The model under review builds one solid part; all positions refer to its coordinate system, in mm. Face numbers are marked on the shaded views. A direction names the side the tool comes from. Round coordinates to 2 decimals unless told otherwise and drop trailing zeros. Order: outer loops, then holes, each group sorted by start corner. A loop starts at its lowest first (then second) coordinate and runs counter-clockwise, first axis right, second up.
1) Machinability: for the marked faces 1, 2 and 3, which of the approach directions +Z, -Z, +X, -X, +Y, -Y give a long, thin tool a straight path to every point of the face, cutting with its end or side? Answer none if there is none.
2) Mouldability with a two-part tool opening along X and no side actions: class the marked faces 4, 5 and 6 as pulls with the +X half, pulls with the -X half, needs draft (parallel to the pull), parting line crosses it, or undercut.
3) Consider section D-D (x = -28.5). Give the boundary of the cut face in (y, z), then the cut area to 3 significant figures.
4) Clearance check with flat-ended pins moving along their axes: P1, Ø1, axis at y = -8, z = -7.5, coming from the +X side (3 decimals); P2, Ø12, axis at x = -48.5, z = -2.5, coming from the +Y side; P3, Ø3.5, axis at y = -9.5, z = -0.5, coming from the -X side (3 decimals). State where each tip first meets the part, or that it passes through.
5) To check wall thickness, follow L1, parallel to X at y = -9.25, z = 2.75 (3 decimals); L2, parallel to X at y = -0.2, z = 0 (3 decimals); L3, parallel to Y at x = 38, z = -1.25. State the ranges of each line that lie inside material, in increasing order.
6) Consider section A-A (z = 0). Give the boundary of the cut face in (x, y) (3 decimals).
7) Consider section B-B (y = -7). Give the boundary of the cut face in (x, z) (3 decimals).
8) Consider section C-C (z = -4.5). Give the boundary of the cut face in (x, y) (3 decimals).
from build123d import *

# Parameters (mm, degrees)
SKETCH1_W          = 82.55
SKETCH1_H          = 25.4
BASE_FLANGE1_DEPTH = 0.7
EDGE_FLANGE1_DEPTH = 25.4
EDGE_FLANGE2_DEPTH = 25.4
EDGE_FLANGE3_DEPTH = 25.4
EDGE_FLANGE4_DEPTH = 25.4
SKETCH19_R         = 2.35
CUT_EXTRUDE1_DEPTH = 59.231440176


# Sheet-metal steps are written as plain solids
with BuildPart() as part:
    # Sketch1 → Base-Flange1 (new body)
    with BuildSketch(Plane(origin=(0, 0, 0), x_dir=(1, 0, 0), z_dir=(0, 1, 0))):
        Rectangle(SKETCH1_W, SKETCH1_H)
    extrude(amount=-BASE_FLANGE1_DEPTH)

    # Edge-Flange1 section (across the edge) → Edge-Flange1 (add)
    with BuildSketch(Plane(origin=(42.275, -0.7, -12.7), x_dir=(-1, 0, 0), z_dir=(0, 0, 1))):
        with BuildLine():
            Line((-0.7, 1), (-0.7, 12))
            Line((-0.7, 12), (0, 12))
            Line((0, 12), (0, 1))
            ThreePointArc((0, 1), (0.292893219, 0.292893219), (1, 0))
            Line((1, 0), (1, -0.7))
            ThreePointArc((1, -0.7), (-0.202081528, -0.202081528), (-0.7, 1))
        make_face()
    extrude(amount=EDGE_FLANGE1_DEPTH)

    # Edge-Flange2 section (across the edge) → Edge-Flange2 (add)
    with BuildSketch(Plane(origin=(42.975, -13.7, 12.7), x_dir=(0, 1, 0), z_dir=(0, 0, -1))):
        with BuildLine():
            Line((-0.7, 1), (-0.7, 12))
            Line((-0.7, 12), (0, 12))
            Line((0, 12), (0, 1))
            ThreePointArc((0, 1), (0.292893219, 0.292893219), (1, 0))
            Line((1, 0), (1, -0.7))
            ThreePointArc((1, -0.7), (-0.202081528, -0.202081528), (-0.7, 1))
        make_face()
    extrude(amount=EDGE_FLANGE2_DEPTH)

    # Edge-Flange3 section (across the edge) → Edge-Flange3 (add)
    with BuildSketch(Plane(origin=(-42.275, -0.7, 12.7), x_dir=(1, 0, 0), z_dir=(0, 0, -1))):
        with BuildLine():
            Line((-0.7, 1), (-0.7, 12))
            Line((-0.7, 12), (0, 12))
            Line((0, 12), (0, 1))
            ThreePointArc((0, 1), (0.292893219, 0.292893219), (1, 0))
            Line((1, 0), (1, -0.7))
            ThreePointArc((1, -0.7), (-0.202081528, -0.202081528), (-0.7, 1))
        make_face()
    extrude(amount=EDGE_FLANGE3_DEPTH)

    # Edge-Flange4 section (across the edge) → Edge-Flange4 (add)
    with BuildSketch(Plane(origin=(-42.975, -13.7, -12.7), x_dir=(0, 1, 0), z_dir=(0, 0, 1))):
        with BuildLine():
            Line((-0.7, 1), (-0.7, 12))
            Line((-0.7, 12), (0, 12))
            Line((0, 12), (0, 1))
            ThreePointArc((0, 1), (0.292893219, 0.292893219), (1, 0))
            Line((1, 0), (1, -0.7))
            ThreePointArc((1, -0.7), (-0.202081528, -0.202081528), (-0.7, 1))
        make_face()
    extrude(amount=EDGE_FLANGE4_DEPTH)

    # Sketch19 → Cut-Extrude1 (cut, through all)
    with BuildSketch(Plane(origin=(0, 0, 0), x_dir=(1, 0, 0), z_dir=(0, 1, 0))):
        with Locations(Location((-33.3248, 0, 0), (0, 0, 270))):
            Circle(SKETCH19_R)
        with Locations(Location((3.175, 0, 0), (0, 0, 270))):
            Circle(SKETCH19_R)
    extrude(amount=-CUT_EXTRUDE1_DEPTH, mode=Mode.SUBTRACT)


solid = part.part
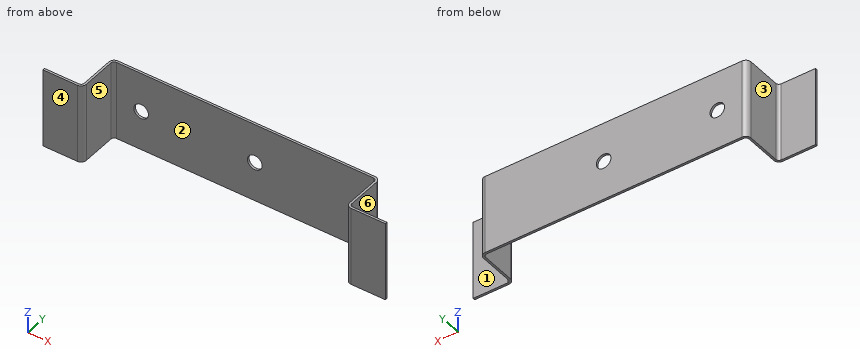
Answer below:
1. face 1: +Z, -Z, +X, +Y
1. face 2: +Z, -Z, -Y
1. face 3: +Z, -Z, -X, +Y
2. face 4: needs draft
2. face 5: undercut
2. face 6: pulls with the +X half
3. outline: (-0.7, -12.7) - (0, -12.7) - (0, 12.7) - (-0.7, 12.7) - close
3. area: 17.8 mm2
4. P1: stops at x = 42.975
4. P2: stops at y = -0.52
4. P3: stops at x = -42.975
5. L1: x = -42.975 to -42.275, 42.275 to 42.975
5. L2: x = -42.075 to -35.675, -30.975 to 0.825, 5.525 to 42.075
5. L3: y = -0.7 to 0
6. outline: (-54.975, -14.4) - (-43.975, -14.4) arc R1.7 ccw to (-42.275, -12.7) - (-42.275, -1.7) arc R1 cw to (-41.275, -0.7) - (-35.675, -0.7) - (-35.675, 0) - (-41.275, 0) arc R1.7 ccw to (-42.975, -1.7) - (-42.975, -12.7) arc R1 cw to (-43.975, -13.7) - (-54.975, -13.7) - close; (-30.975, -0.7) - (0.825, -0.7) - (0.825, 0) - (-30.975, 0) - close; (5.525, -0.7) - (41.275, -0.7) arc R1 cw to (42.275, -1.7) - (42.275, -12.7) arc R1.7 ccw to (43.975, -14.4) - (54.975, -14.4) - (54.975, -13.7) - (43.975, -13.7) arc R1 cw to (42.975, -12.7) - (42.975, -1.7) arc R1.7 ccw to (41.275, 0) - (5.525, 0) - close
7. outline: (-42.975, -12.7) - (-42.275, -12.7) - (-42.275, 12.7) - (-42.975, 12.7) - close; (42.275, -12.7) - (42.975, -12.7) - (42.975, 12.7) - (42.275, 12.7) - close
8. outline: (-54.975, -14.4) - (-43.975, -14.4) arc R1.7 ccw to (-42.275, -12.7) - (-42.275, -1.7) arc R1 cw to (-41.275, -0.7) - (41.275, -0.7) arc R1 cw to (42.275, -1.7) - (42.275, -12.7) arc R1.7 ccw to (43.975, -14.4) - (54.975, -14.4) - (54.975, -13.7) - (43.975, -13.7) arc R1 cw to (42.975, -12.7) - (42.975, -1.7) arc R1.7 ccw to (41.275, 0) - (-41.275, 0) arc R1.7 ccw to (-42.975, -1.7) - (-42.975, -12.7) arc R1 cw to (-43.975, -13.7) - (-54.975, -13.7) - close
